from build123d import *

# Parameters (mm, degrees)
SKETCH1_R               = 6
SKETCH1_R_2             = 1.9
BOSS_EXTRUDE1_DEPTH     = 6
SKETCH2_R               = 6
SKETCH2_R_2             = 2.55
BOSS_EXTRUDE2_DEPTH     = 11
SKETCH3_R               = 2.55
BOSS_EXTRUDE3_DEPTH     = 17
BOSS_EXTRUDE4_DEPTH     = 30.75
BOSS_EXTRUDE6_DEPTH     = 13.75
CUT_EXTRUDE1_DEPTH      = 26
CUT_EXTRUDE2_DEPTH      = 59.698913959
FILLET1_R               = 2
FILLET2_R               = 2
CUT_EXTRUDE3_DEPTH      = 3
CUT_EXTRUDE4_DEPTH      = 59.698913959
CUT_EXTRUDE4_DEPTH_BACK = 26
SKETCH12_W              = 5
SKETCH12_H              = 34.4
FILLET3_R               = 0.5


with BuildPart() as part:
    # Sketch1 → Boss-Extrude1 (new body)
    with BuildSketch(Plane.XY):
        Circle(SKETCH1_R)
        Circle(SKETCH1_R_2, mode=Mode.SUBTRACT)
    extrude(amount=BOSS_EXTRUDE1_DEPTH)

    # Sketch2 → Boss-Extrude2 (add)
    with BuildSketch(Plane.XY.offset(6)):
        Circle(SKETCH2_R)
        Circle(SKETCH2_R_2, mode=Mode.SUBTRACT)
    extrude(amount=BOSS_EXTRUDE2_DEPTH)

    # Sketch3 → Boss-Extrude3 (add)
    with BuildSketch(Plane(origin=(0, 0, 0), x_dir=(-1, 0, 0), z_dir=(0, 0, -1))):
        with BuildLine():
            Line((-6, 0), (-6, -16))
            Line((-6, -16), (6, -16))
            Line((6, -16), (6, 0))
            ThreePointArc((6, 0), (0, 6), (-6, 0))
        make_face()
        with Locations(Location((0, 0, 0), (0, 0, 180))):
            Circle(SKETCH3_R, mode=Mode.SUBTRACT)
    extrude(amount=-BOSS_EXTRUDE3_DEPTH)

    # Sketch4 → Boss-Extrude4 (add)
    with BuildSketch(Plane(origin=(0, 0, 0), x_dir=(-1, 0, 0), z_dir=(0, 0, -1))):
        Polygon((-6, -16), (-6, -8), (-14, -8), (-14, -48), (14, -48), (14, -8), (6, -8), (6, -16), align=None)
    extrude(amount=-BOSS_EXTRUDE4_DEPTH)

    # Sketch9 → Boss-Extrude6 (add)
    with BuildSketch(Plane.XY.offset(17)):
        Polygon((-6, -8), (-4, -8), (-4, -14), (4, -14), (4, -8), (6, -8), (6, -16), (-6, -16), align=None)
    extrude(amount=BOSS_EXTRUDE6_DEPTH)

    # Sketch5 → Cut-Extrude1 (cut)
    with BuildSketch(Plane(origin=(0, 0, 0), x_dir=(-1, 0, 0), z_dir=(0, 0, -1))):
        with BuildLine():
            Line((-5.8, -14), (-5.8, -42))
            ThreePointArc((-5.8, -42), (-9, -45.2), (-12.2, -42))
            Line((-12.2, -42), (-12.2, -14))
            ThreePointArc((-12.2, -14), (-9, -10.8), (-5.8, -14))
        make_face()
        with BuildLine():
            Line((5.8, -14), (5.8, -42))
            ThreePointArc((5.8, -42), (9, -45.2), (12.2, -42))
            Line((12.2, -42), (12.2, -14))
            ThreePointArc((12.2, -14), (9, -10.8), (5.8, -14))
        make_face()
    extrude(amount=-CUT_EXTRUDE1_DEPTH, mode=Mode.SUBTRACT)

    # Sketch7 → Cut-Extrude2 (cut, through all)
    with BuildSketch(Plane(origin=(0, 0, 0), x_dir=(-1, 0, 0), z_dir=(0, 0, -1))):
        with BuildLine():
            Line((-7.4, -14), (-7.4, -42))
            ThreePointArc((-7.4, -42), (-9, -43.6), (-10.6, -42))
            Line((-10.6, -42), (-10.6, -14))
            ThreePointArc((-10.6, -14), (-9, -12.4), (-7.4, -14))
        make_face()
        with BuildLine():
            Line((7.4, -14), (7.4, -42))
            ThreePointArc((7.4, -42), (9, -43.6), (10.6, -42))
            Line((10.6, -42), (10.6, -14))
            ThreePointArc((10.6, -14), (9, -12.4), (7.4, -14))
        make_face()
    extrude(amount=-CUT_EXTRUDE2_DEPTH, mode=Mode.SUBTRACT)

    # Fillet1
    fillet1_edges = [part.edges().sort_by_distance(p)[0] for p in [
        (6, -8, 8.5),
        (-6, -8, 8.5),
        (-14, -8, 15.375),
        (-14, -48, 15.375),
        (14, -48, 15.375),
        (14, -8, 15.375),
    ]]
    fillet(fillet1_edges, radius=FILLET1_R)

    # Fillet2
    fillet2_edges = [part.edges().sort_by_distance(p)[0] for p in [
        (-4, -8, 23.875),
        (-4, -14, 23.875),
        (4, -14, 23.875),
        (4, -8, 23.875),
    ]]
    fillet(fillet2_edges, radius=FILLET2_R)

    # Sketch10 → Cut-Extrude3 (cut)
    with BuildSketch(Plane(origin=(0, 0, 0), x_dir=(-1, 0, 0), z_dir=(0, 0, -1))):
        Polygon((0, 3.348631561), (-2.9, 1.674315781), (-2.9, -1.674315781), (0, -3.348631561), (2.9, -1.674315781), (2.9, 1.674315781), align=None)
    extrude(amount=-CUT_EXTRUDE3_DEPTH, mode=Mode.SUBTRACT)

    # Sketch12 → Cut-Extrude4 (cut, two sides: drawn at the far end of the back side and taken through both)
    with BuildSketch(Plane(origin=(0, 0, 0), x_dir=(-1, 0, 0), z_dir=(0, 0, -1)).offset(-CUT_EXTRUDE4_DEPTH_BACK)):
        with Locations((-11.5, -28)):
            Rectangle(SKETCH12_W, SKETCH12_H)
        with Locations((11.5, -28)):
            Rectangle(SKETCH12_W, SKETCH12_H)
    extrude(amount=CUT_EXTRUDE4_DEPTH + CUT_EXTRUDE4_DEPTH_BACK, mode=Mode.SUBTRACT)

    # Fillet3
    fillet3_edges = [part.edges().sort_by_distance(p)[0] for p in [
        (10, -8, 0),
        (-10, -8, 0),
        (-6, -3, 0),
        (0, -48, 0),
        (14, -10.4, 0),
        (-14, -45.6, 0),
        (13.414213562, -8.585786438, 0),
        (13.414213562, -47.414213562, 0),
        (-13.414213562, -8.585786438, 0),
        (-13.414213562, -47.414213562, 0),
        (6.585786438, -7.414213562, 0),
        (-6.585786438, -7.414213562, 0),
        (0, 6, 0),
        (6, -3, 0),
        (-1.45, 2.511473671, 0),
        (1.45, 2.511473671, 0),
        (2.9, 0, 0),
        (1.45, -2.511473671, 0),
        (-1.45, -2.511473671, 0),
        (-2.9, 0, 0),
        (6.7372583, -44.2627417, 0),
        (-6.7372583, -11.7372583, 0),
        (14, -45.6, 0),
        (-14, -10.4, 0),
        (14, -45.2, 13),
        (11.5, -45.2, 0),
        (14, -10.8, 13),
        (11.5, -10.8, 0),
        (-14, -10.8, 13),
        (-11.5, -10.8, 0),
        (-14, -45.2, 13),
        (-11.5, -45.2, 0),
        (6.7372583, -11.7372583, 0),
        (5.8, -28, 0),
        (-5.8, -28, 0),
        (-6.7372583, -44.2627417, 0),
    ]]
    fillet(fillet3_edges, radius=FILLET3_R)


solid = part.part
Here's how the part is built. I have some questions about the finished solid (model axes, mm). A direction names the side the tool comes from. Coordinates: 2 decimals unless noted, no trailing zeros. Loops run counter-clockwise (first coordinate to the right, second up) from the corner with the lowest first, then second, coordinate; pieces in that order, holes last.
1. Imagine slicing it at D-D, the plane y = -5. Please give me the cut outline in (x, z), and give its area (3 significant figures).
2. I need wall thicknesses on L1, parallel to X at y = 0, z = 5; L2, parallel to Y at x = 10, z = 9; L3, parallel to Y at x = 0, z = 9.5. Which ranges of each line are inside material? Lowest first, please.
3. Imagine slicing it at B-B, the plane y = -31. Please give me the cut outline in (x, z), and give its area (3 significant figures).
4. For faces 4 (the flat face through (11, -10.8, 13)), 5 (the flat face through (1.43, 2.523, 1.732)), 6 (the cylindrical face through (4.6, -8.57, 23.97)), 7 (the cylindrical face through (9, -12.4, 28.3)), which set-ups out of +Z, -Z, +X, -X, +Y, -Y let a thin tool reach every point of the face, with its end or its side?
5. If we mould it in two halves opening along Y, with no side actions, what happens to faces 1 (the flat face through (6, -3, 9)), 2 (the cylindrical face through (6.713, -44.238, 13.072)), 3 (the flat face through (0, -48, 15))? For each: pulls with the +Y half, pulls with the -Y half, needs draft (parallel to the pull), parting line crosses it, or undercut.
6. For P1, Ø6.5, axis at y = -4, z = 13, coming from the -X side; P2, Ø0.8, axis at y = 0, z = 2, coming from the +X side; P3, Ø5.5, axis at x = -1, y = -0.5, coming from the +Z side, each with a flat end and sliding along its axis, tell me the tip position at first contact or that it passes through.
Taken from the geometry:
1. outline: (-6, 0.5) arc R0.5 ccw to (-5.5, 0) - (5.5, 0) arc R0.5 ccw to (6, 0.5) - (6, 17) - (-6, 17) - close
1. area: 204 mm2
2. L1: x = -6 to -1.9, 1.9 to 6
2. L2: y = -48 to -45.2, -10.8 to -8
2. L3: y = -48 to -2.55, 2.55 to 6
3. outline: (-14, 26) - (-10.6, 26) - (-10.6, 30.75) - (-14, 30.75) - close; (-7.4, 26) - (-5.8, 26) - (-5.8, 0.5) arc R0.5 ccw to (-5.3, 0) - (5.3, 0) arc R0.5 ccw to (5.8, 0.5) - (5.8, 26) - (7.4, 26) - (7.4, 30.75) - (-7.4, 30.75) - close; (10.6, 26) - (14, 26) - (14, 30.75) - (10.6, 30.75) - close
3. area: 404 mm2
4. face 4: -Z, +X
4. face 5: -Z
4. face 6: +Z, +Y
4. face 7: +Z, -Z
5. face 1: needs draft
5. face 2: undercut
5. face 3: pulls with the -Y half
6. P1: stops at x = -6.44
6. P2: stops at x = 6
6. P3: stops at z = 17
